```python
from build123d import *

# Parameters (mm, degrees)
SKETCH1_W               = 85.725
SKETCH1_H               = 85.725
SKETCH1_R               = 24.511
BOSS_EXTRUDE1_DEPTH     = 25.4
SKETCH2_R               = 3.572453457
CUT_EXTRUDE1_DEPTH      = 26.4
MIRROR2_COPY_1_SKETCH_R = 3.572453457
MIRROR2_COPY_1_DEPTH    = 26.4
SKETCH3_W               = 78.105
SKETCH3_H               = 78.105
CUT_EXTRUDE2_DEPTH      = 22.225
FILLET1_R               = 2.54
SKETCH5_R               = 34.925
SKETCH5_R_2             = 32.258
CUT_EXTRUDE4_DEPTH      = 1.27
SKETCH6_W               = 10.16
SKETCH6_H               = 11.43
CUT_EXTRUDE5_DEPTH      = 26.4
FILLET2_R               = 1.27
SKETCH7_R               = 28.6131
CUT_EXTRUDE6_DEPTH      = 0.635


with BuildPart() as part:
    # Sketch1 → Boss-Extrude1 (new body)
    with BuildSketch(Plane.XY):
        Rectangle(SKETCH1_W, SKETCH1_H)
        Circle(SKETCH1_R, mode=Mode.SUBTRACT)
    extrude(amount=BOSS_EXTRUDE1_DEPTH)

    # Sketch2 → Cut-Extrude1 (cut, through all)
    with BuildSketch(Plane.XY.offset(25.4)):
        with Locations((-31.75, 31.75)):
            Circle(SKETCH2_R)
    cut_extrude1 = extrude(amount=-CUT_EXTRUDE1_DEPTH, mode=Mode.SUBTRACT)

    # Mirror1: Cut-Extrude1 across plane
    add(cut_extrude1.mirror(Plane(origin=(0, 0, 0), x_dir=(0, 0, 1), z_dir=(1, 0, 0))), mode=Mode.SUBTRACT)

    # Mirror2: Cut-Extrude1 across plane
    add(cut_extrude1.mirror(Plane.ZX), mode=Mode.SUBTRACT)

    # Mirror2 copy 1 sketch → Mirror2 copy 1 (cut, through all)
    with BuildSketch(Plane(origin=(0, 0, 25.4), x_dir=(-1, 0, 0), z_dir=(0, 0, 1))):
        with Locations((-31.75, 31.75)):
            Circle(MIRROR2_COPY_1_SKETCH_R)
    extrude(amount=-MIRROR2_COPY_1_DEPTH, mode=Mode.SUBTRACT)

    # Sketch3 → Cut-Extrude2 (cut)
    with BuildSketch(Plane(origin=(0, 0, 0), x_dir=(-1, 0, 0), z_dir=(0, 0, -1))):
        Rectangle(SKETCH3_W, SKETCH3_H)
    extrude(amount=-CUT_EXTRUDE2_DEPTH, mode=Mode.SUBTRACT)

    # Fillet1
    fillet1_edges = [part.edges().sort_by_distance(p)[0] for p in [
        (-39.0525, -39.0525, 11.1125),
        (-39.0525, 39.0525, 11.1125),
        (39.0525, 39.0525, 11.1125),
        (39.0525, -39.0525, 11.1125),
        (-42.8625, 42.8625, 12.7),
        (42.8625, 42.8625, 12.7),
        (42.8625, -42.8625, 12.7),
        (-42.8625, -42.8625, 12.7),
    ]]
    fillet(fillet1_edges, radius=FILLET1_R)

    # Sketch5 → Cut-Extrude4 (cut)
    with BuildSketch(Plane.XY.offset(25.4)):
        Circle(SKETCH5_R)
        Circle(SKETCH5_R_2, mode=Mode.SUBTRACT)
    extrude(amount=-CUT_EXTRUDE4_DEPTH, mode=Mode.SUBTRACT)

    # Sketch6 → Cut-Extrude5 (cut, through all)
    with BuildSketch(Plane.XY.offset(25.4)):
        with Locations((0, 24.765)):
            Rectangle(SKETCH6_W, SKETCH6_H)
    extrude(amount=-CUT_EXTRUDE5_DEPTH, mode=Mode.SUBTRACT)

    # Fillet2
    fillet2_edges = [part.edges().sort_by_distance(p)[0] for p in [
        (-5.08, 30.48, 23.8125),
        (5.08, 30.48, 23.8125),
    ]]
    fillet(fillet2_edges, radius=FILLET2_R)

    # Sketch7 → Cut-Extrude6 (cut)
    with BuildSketch(Plane(origin=(0, 0, 22.225), x_dir=(-1, 0, 0), z_dir=(0, 0, -1))):
        Circle(SKETCH7_R)
    extrude(amount=-CUT_EXTRUDE6_DEPTH, mode=Mode.SUBTRACT)


solid = part.part
```
Model file for the job. Use its own axes, mm. A direction names the side the tool comes from. Coordinates: 2 decimals unless noted, no trailing zeros. Order: outer loops, then holes, each group sorted by start corner. A loop starts at its lowest first (then second) coordinate and runs counter-clockwise, first axis right, second up. Notation, with made-up numbers: (-8.5, 63.25) -> (5.5, 63.25) arc R13 ccw to (5.5, 83.25) -> close; hole circle Ø6 at (67, -31.5). An arc over 180 degrees is marked (long way). Answer as a JSON object with one key per item and string values. Group by question number.
1) Drill centre lines: L1, parallel to X at y = -31.75, z = 23.6; L2, parallel to Y at x = -10.5, z = 9.5. Where is each one in solid material? Low to high.
2) Cut at A-A, the plane y = 0. Write the cut outline in (x, z) (1 decimal).
3) Cut at D-D, the plane x = 14. Write the cut outline in (y, z) (1 decimal).
4) Which spindle directions (+Z, -Z, +X, -X, +Y, -Y) get a long thin tool onto all of the face, cutting with end or side? Do faces 5 (the face through (5.08, 27, 24)), 6 (the face through (1, 39.052, 11)), 7 (the face through (-1, -42.862, 13)), 8 (the face through (31, -10, 24.13)). Say none if no direction does.
5) Flat gauge pins, fed straight in: pin 1 (4 mm diameter, centred on x = -6, y = 27.5, fed in from -Z) (3 decimals); pin 2 (5.5 mm diameter, centred on x = -31.75, y = -31.75, fed in from -Z); pin 3 (1.5 mm diameter, centred on x = -18.5, y = -28, fed in from +Z). Where does each tip first touch, or does it go through?
6) Cut at B-B, the plane x = 0. Write the cut outline in (y, z) (1 decimal), then the cut area to 3 significant figures.
7) Cut at C-C, the plane z = 5. Write the cut outline in (x, y), then the cut area to 3 significant figures.
8) Pull direction X, two halves, no side cores. Call faces 1 (the face through (42.099, -42.138, 12.878)), 2 (the face through (-28.34, -32.82, 23.83)), 3 (the face through (-39.052, -1, 11)), 4 (the face through (-3, -41, 0)): +X half, -X half, draft (parallel to the pull), parting line (faces both ways), or undercut.
Check values:
{
 "1": {"L1": "x = -42.86 to -35.32, -28.18 to 28.18, 35.32 to 42.86", "L2": "y = -42.86 to -39.05, 39.05 to 42.86"},
 "2": {"outline": "(-42.9, 0) -> (-39.1, 0) -> (-39.1, 22.2) -> (-28.6, 22.2) -> (-28.6, 22.9) -> (-24.5, 22.9) -> (-24.5, 25.4) -> (-32.3, 25.4) -> (-32.3, 24.1) -> (-34.9, 24.1) -> (-34.9, 25.4) -> (-42.9, 25.4) -> close; (24.5, 22.9) -> (28.6, 22.9) -> (28.6, 22.2) -> (39.1, 22.2) -> (39.1, 0) -> (42.9, 0) -> (42.9, 25.4) -> (34.9, 25.4) -> (34.9, 24.1) -> (32.3, 24.1) -> (32.3, 25.4) -> (24.5, 25.4) -> close"},
 "3": {"outline": "(-42.9, 0) -> (-39.1, 0) -> (-39.1, 22.2) -> (-25, 22.2) -> (-25, 22.9) -> (-20.1, 22.9) -> (-20.1, 25.4) -> (-29.1, 25.4) -> (-29.1, 24.1) -> (-32, 24.1) -> (-32, 25.4) -> (-42.9, 25.4) -> close; (20.1, 22.9) -> (25, 22.9) -> (25, 22.2) -> (39.1, 22.2) -> (39.1, 0) -> (42.9, 0) -> (42.9, 25.4) -> (32, 25.4) -> (32, 24.1) -> (29.1, 24.1) -> (29.1, 25.4) -> (20.1, 25.4) -> close"},
 "4": {"face 5": "+Z, -Z", "face 6": "-Z", "face 7": "+Z, -Z, +X, -X, -Y", "face 8": "+Z"},
 "5": {"pin 1": "stops at z = 22.225", "pin 2": "passes through", "pin 3": "stops at z = 24.13"},
 "6": {"outline": "(-42.9, 0) -> (-39.1, 0) -> (-39.1, 22.2) -> (-28.6, 22.2) -> (-28.6, 22.9) -> (-24.5, 22.9) -> (-24.5, 25.4) -> (-32.3, 25.4) -> (-32.3, 24.1) -> (-34.9, 24.1) -> (-34.9, 25.4) -> (-42.9, 25.4) -> close; (30.5, 22.2) -> (39.1, 22.2) -> (39.1, 0) -> (42.9, 0) -> (42.9, 25.4) -> (34.9, 25.4) -> (34.9, 24.1) -> (32.3, 24.1) -> (32.3, 25.4) -> (30.5, 25.4) -> close", "area": "258 mm²"},
 "7": {"outline": "(-42.86, -40.32) arc R2.54 ccw to (-40.32, -42.86) -> (40.32, -42.86) arc R2.54 ccw to (42.86, -40.32) -> (42.86, 40.32) arc R2.54 ccw to (40.32, 42.86) -> (-40.32, 42.86) arc R2.54 ccw to (-42.86, 40.32) -> close; hole (-39.05, -36.51) arc R2.54 ccw to (-36.51, -39.05) -> (36.51, -39.05) arc R2.54 ccw to (39.05, -36.51) -> (39.05, 36.51) arc R2.54 ccw to (36.51, 39.05) -> (-36.51, 39.05) arc R2.54 ccw to (-39.05, 36.51) -> close", "area": "1,250 mm²"},
 "8": {"face 1": "+X half", "face 2": "undercut", "face 3": "undercut", "face 4": "draft"}
}
